Input: part model. Units: mm. Frame: model coordinates. Face numbers are marked on the shaded views. A direction names the side the tool comes from. Round coordinates to 2 decimals unless told otherwise and drop trailing zeros. Loops run counter-clockwise (first coordinate to the right, second up) from the corner with the lowest first, then second, coordinate; pieces in that order, holes last.
1) Section A-A, the plane y = 0. Return loops of the section in (x, z).
2) Section B-B, the plane x = 7. Return loops of the section in (y, z).
3) Draft query along Y for the marked faces 1, 2 and 3. Return one class per face: pulls with the +Y half, pulls with the -Y half, needs draft (parallel to the pull), parting line crosses it, or undercut.
4) Section D-D, the plane z = 18. Return loops of the section in (x, y).
5) Access query for the marked faces 4, 5 and 6. Directions: +Z, -Z, +X, -X, +Y, -Y. A direction counts if a zero-diameter tool reaches every point of the face in a straight line with its end or side. Return the directions, or none.
6) Section C-C, the plane z = 12.25. Return loops of the section in (x, y).
7) First-contact query: pin 1 (6 mm diameter, centred on x = 5, z = 13.5, fed in from +Y); pin 2 (12 mm diameter, centred on y = -32, z = 2, fed in from -X); pin 3 (3 mm diameter, centred on y = -30, z = 14, fed in from -X). Flat tips, straight axial feed; report the tip coordinate or a pass-through.
8) Ray query, line 1 along Y through (x, z) = (0, 9.25); line 2 along Z through (x, y) = (-5, -9.5); line 3 along Y through (x, z) = (2, 6.75). Return the intervals inside material, ascending.
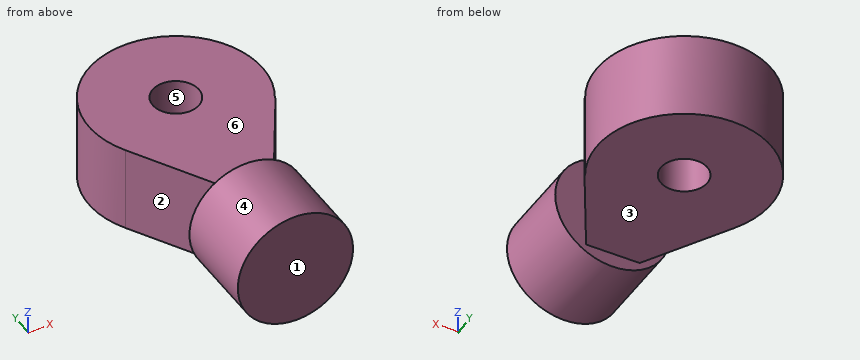
Autodesk Inventor part; units mm, degrees
ref_plane "YZ Plane" through (0, 0, 0) normal (1, 0, 0) x (0, 1, 0)
ref_plane "XZ Plane" through (0, 0, 0) normal (0, 1, 0) x (-1, 0, 0)
ref_plane "XY Plane" through (0, 0, 0) normal (0, 0, 1) x (1, 0, 0)
sketch "Sketch1" plane through (0, 0, 0) normal (0, 0, 1) x (1, 0, 0)
  arc A0 (16.5296, -9.4696) -> (-16.4657, -9.5803) centre (0, 0) ccw
  circle A1 centre (0, 0) radius 5.08
  line L0 (16.5296, -9.4696) -> (16.6574, -9.4696)
  line L1 (16.6574, -9.4696) -> (5.9637, -27.9917)
  line L2 (-5.8359, -27.9917) -> (-16.5296, -9.4696)
  line L3 (-5.8359, -27.9917) -> (5.9637, -27.9917)
  point P0 (0.0639, -19.0499)
  dimension "d0" = 38.1
  dimension "d1" = 10.16
extrude "Extrusion1" add sketch "Sketch1" along normal blind 19.05
sketch "Sketch2" plane through (-5.8359, -27.9917, 0) normal (0, -1, 0) x (1, 0, 0)
  circle A0 centre (5.8941, 9.525) radius 12.7
  line L0 (11.7996, 0) -> (11.7996, 19.05)
  line L1 (0, 0) -> (11.7996, 0)
  point P0 (5.8359, 0)
  dimension "d4" = 25.4
  dimension "d5" = 5.9055
  dimension "d6" = 9.525
extrude "Extrusion2" add sketch "Sketch2" along normal blind 19.05
properties part number "Load Notch Insert"
Final values:
1. outline: (-19.05, 0) - (-5.08, 0) - (-5.08, 19.05) - (-19.05, 19.05) - close; (5.08, 0) - (19.05, 0) - (19.05, 19.05) - (5.08, 19.05) - close
2. outline: (-47.04, -1.11) - (-27.99, -1.11) - (-27.99, 20.16) - (-47.04, 20.16) - close; (-26.2, 0) - (17.72, 0) - (17.72, 19.05) - (-26.2, 19.05) - close
3. face 1: pulls with the -Y half
3. face 2: undercut
3. face 3: needs draft
4. outline: (-16.47, -9.58) - (-5.84, -27.99) - (-9.4, -27.99) - (-9.4, -47.04) - (9.52, -47.04) - (9.52, -27.99) - (5.96, -27.99) - (16.66, -9.47) - (16.53, -9.47) arc R19.05 ccw (long way) to start; hole circle Ø10.16 at (0, 0)
5. face 4: -Y
5. face 5: +Z, -Z
5. face 6: +Z, +X, -X, +Y
6. outline: (-16.47, -9.58) - (-5.84, -27.99) - (-12.35, -27.99) - (-12.35, -47.04) - (12.46, -47.04) - (12.46, -27.99) - (5.96, -27.99) - (16.66, -9.47) - (16.53, -9.47) arc R19.05 ccw (long way) to start; hole circle Ø10.16 at (0, 0)
7. pin 1: stops at y = 18.94
7. pin 2: stops at x = -12.55
7. pin 3: stops at x = -12.29
8. line 1: y = -47.04 to -5.08, 5.08 to 19.05
8. line 2: z = 0 to 19.05
8. line 3: y = -47.04 to -4.67, 4.67 to 18.94
